from build123d import *

# Parameters (mm, degrees)
SKETCH1_R           = 6
SKETCH1_R_2         = 2.5
BOSS_EXTRUDE1_DEPTH = 4.5
SKETCH2_R           = 4.25
CUT_EXTRUDE1_DEPTH  = 1.5
BOSS_EXTRUDE2_START = 10
SKETCH3_R           = 30
BOSS_EXTRUDE2_DEPTH = 10
SKETCH4_R           = 2.1
CUT_EXTRUDE2_DEPTH  = 43


with BuildPart() as part:
    # Sketch1 → Boss-Extrude1 (new body)
    # profile 1 of 4: a face of its own
    with BuildSketch(Plane(origin=(0, 0, 0), x_dir=(1, 0, 0), z_dir=(0, 1, 0))):
        with BuildLine():
            ThreePointArc((0, 30), (-12.247448714, 27.386127875), (-22.360679775, 20))
            ThreePointArc((-22.360679775, 20), (-10.704662693, -28.025170769), (30, 0))
            ThreePointArc((30, 0), (28.025170769, 10.704662693), (22.360679775, 20))
            ThreePointArc((22.360679775, 20), (12.247448714, 27.386127875), (0, 30))
        make_face()
    # profile 2 of 4: a face of its own
    with BuildSketch(Plane(origin=(0, 0, 0), x_dir=(1, 0, 0), z_dir=(0, 1, 0))):
        with BuildLine():
            Line((22.360679775, 20), (4.472135955, 40))
            ThreePointArc((4.472135955, 40), (5.605034154, 38.140932539), (6, 36))
            ThreePointArc((6, 36), (4.242640687, 31.757359313), (0, 30))
            ThreePointArc((0, 30), (12.247448714, 27.386127875), (22.360679775, 20))
        make_face()
    # profile 3 of 4: a face of its own
    with BuildSketch(Plane(origin=(0, 0, 0), x_dir=(1, 0, 0), z_dir=(0, 1, 0))):
        with BuildLine():
            ThreePointArc((0, 30), (-5.477225575, 33.550510257), (-4.472135955, 40))
            Line((-4.472135955, 40), (-22.360679775, 20))
            ThreePointArc((-22.360679775, 20), (-12.247448714, 27.386127875), (0, 30))
        make_face()
    # profile 4 of 4: a face of its own
    with BuildSketch(Plane(origin=(0, 0, 0), x_dir=(1, 0, 0), z_dir=(0, 1, 0))):
        with Locations((0, 36)):
            Circle(SKETCH1_R)
        with Locations(Location((0, 36, 0), (0, 0, 270))):
            Circle(SKETCH1_R_2, mode=Mode.SUBTRACT)
    extrude(amount=BOSS_EXTRUDE1_DEPTH)

    # Sketch2 → Cut-Extrude1 (cut)
    with BuildSketch(Plane(origin=(0, 4.5, 0), x_dir=(1, 0, 0), z_dir=(0, 1, 0))):
        with Locations(Location((0, 23, 0), (0, 0, 270))):
            Circle(SKETCH2_R)
        with Locations(Location((19.918584287, 11.5, 0), (0, 0, 270))):
            Circle(SKETCH2_R)
        with Locations(Location((19.918584287, -11.5, 0), (0, 0, 270))):
            Circle(SKETCH2_R)
        with Locations(Location((0, -23, 0), (0, 0, 270))):
            Circle(SKETCH2_R)
        with Locations(Location((-19.918584287, -11.5, 0), (0, 0, 270))):
            Circle(SKETCH2_R)
        with Locations(Location((-19.918584287, 11.5, 0), (0, 0, 270))):
            Circle(SKETCH2_R)
    extrude(amount=-CUT_EXTRUDE1_DEPTH, mode=Mode.SUBTRACT)

    # Sketch3 → Boss-Extrude2 (add)
    with BuildSketch(Plane.XZ.offset(BOSS_EXTRUDE2_START)):
        with Locations(Location((0, 0, 0), (0, 0, 270))):
            Circle(SKETCH3_R)
    extrude(amount=-BOSS_EXTRUDE2_DEPTH)

    # Sketch4 → Cut-Extrude2 (cut)
    with BuildSketch(Plane(origin=(0, 4.5, 0), x_dir=(1, 0, 0), z_dir=(0, 1, 0))):
        with Locations(Location((0, 23, 0), (0, 0, 270))):
            Circle(SKETCH4_R)
        with Locations(Location((19.918584287, 11.5, 0), (0, 0, 270))):
            Circle(SKETCH4_R)
        with Locations(Location((19.918584287, -11.5, 0), (0, 0, 270))):
            Circle(SKETCH4_R)
        with Locations(Location((0, -23, 0), (0, 0, 270))):
            Circle(SKETCH4_R)
        with Locations(Location((-19.918584287, -11.5, 0), (0, 0, 270))):
            Circle(SKETCH4_R)
        with Locations(Location((-19.918584287, 11.5, 0), (0, 0, 270))):
            Circle(SKETCH4_R)
    extrude(amount=-CUT_EXTRUDE2_DEPTH, mode=Mode.SUBTRACT)


solid = part.part
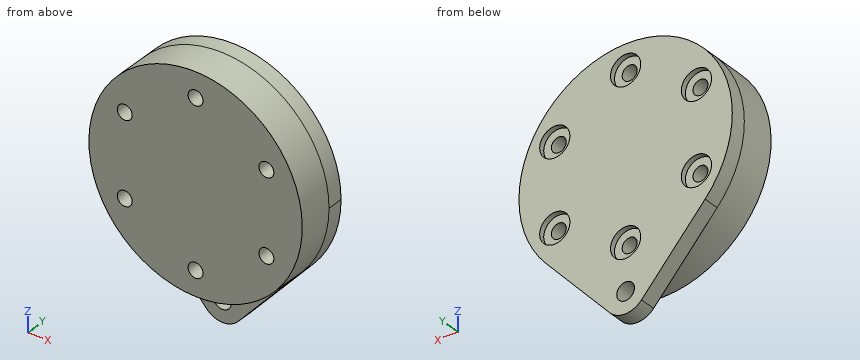
Can you work these out from the model? Positions are in its coordinate system, mm. Round coordinates to 2 decimals unless told otherwise and drop trailing zeros. Write each loop counter-clockwise with the first axis right and the second up, starting at its lowest first coordinate (ties: lowest second). Pieces come first, ordered by that corner, then holes. Notation, with made-up numbers: (68, 75) -> (114, 75) arc R14 ccw to (114, 80) -> close; hole circle Ø4 at (-39, -39.5). An arc over 180 degrees is marked (long way). One line per question, with ' | ' between items. Start each with the question number.
1) I'm going to push flat-ended pins straight in: P1, Ø8, axis at x = 16, y = -3, coming from the +Z side; P2, Ø2, axis at y = -6.5, z = -25, coming from the +X side; P3, Ø2.5, axis at x = 0, z = -25, coming from the +Y side. Where does each tip first touch, or does it pass through?
2) Suppose I cut it at B-B on z = 23. Write out the boundary of the cut face in (x, y), then the cut area to 3 significant figures.
3) Suppose I cut it at C-C on x = -21. Write out the boundary of the cut face in (y, z).
4) Suppose I cut it at D-D on y = -8. Write out the boundary of the cut face in (x, z), then the cut area to 3 significant figures.
5) Suppose I cut it at A-A on x = 0. Write out the boundary of the cut face in (y, z).
6) I need wall thicknesses on line 1 (Z direction, x = 20, y = -1); line 2 (X direction, y = -8.5, z = -13); line 3 (X direction, y = -6.5, z = 11.5). Which ranges of each line are inside material? Lowest first, please. Write a range as [from, to].
Return value:
1) P1: stops at z = 27.5 | P2: stops at x = 18 | P3: stops at y = 3
2) outline: (-19.26, -10) -> (-2.1, -10) -> (-2.1, 3) -> (-4.25, 3) -> (-4.25, 4.5) -> (-19.26, 4.5) -> close; (2.1, -10) -> (19.26, -10) -> (19.26, 4.5) -> (4.25, 4.5) -> (4.25, 3) -> (2.1, 3) -> close | area: 491 mm2
3) outline: (-10, -21.42) -> (0, -21.42) -> (0, -21.52) -> (4.5, -21.52) -> (4.5, -15.61) -> (3, -15.61) -> (3, -13.3) -> (-10, -13.3) -> close; (-10, -9.7) -> (3, -9.7) -> (3, -7.39) -> (4.5, -7.39) -> (4.5, 7.39) -> (3, 7.39) -> (3, 9.7) -> (-10, 9.7) -> close; (-10, 13.3) -> (3, 13.3) -> (3, 15.61) -> (4.5, 15.61) -> (4.5, 21.42) -> (-10, 21.42) -> close
4) outline: circle Ø60 at (0, 0); hole circle Ø4.2 at (-19.92, -11.5); hole circle Ø4.2 at (-19.92, 11.5); hole circle Ø4.2 at (0, -23); hole circle Ø4.2 at (0, 23); hole circle Ø4.2 at (19.92, -11.5); hole circle Ø4.2 at (19.92, 11.5) | area: 2,740 mm2
5) outline: (-10, -30) -> (0, -30) -> (0, -33.5) -> (4.5, -33.5) -> (4.5, -27.25) -> (3, -27.25) -> (3, -25.1) -> (-10, -25.1) -> close; (-10, -20.9) -> (3, -20.9) -> (3, -18.75) -> (4.5, -18.75) -> (4.5, 18.75) -> (3, 18.75) -> (3, 20.9) -> (-10, 20.9) -> close; (-10, 25.1) -> (3, 25.1) -> (3, 27.25) -> (4.5, 27.25) -> (4.5, 30) -> (-10, 30) -> close; (0, -42) -> (4.5, -42) -> (4.5, -38.5) -> (0, -38.5) -> close
6) line 1: z = [-22.36, -13.6], [-9.4, 9.4], [13.6, 22.36] | line 2: x = [-27.04, -21.39], [-18.45, 18.45], [21.39, 27.04] | line 3: x = [-27.71, -22.02], [-17.82, 17.82], [22.02, 27.71]
